Could you check a few things on this model? Use its own coordinates, in mm. A direction names the side the tool comes from. Coordinates: 2 decimals unless noted, no trailing zeros. Write each loop counter-clockwise with the first axis right and the second up, starting at its lowest first coordinate (ties: lowest second). Pieces come first, ordered by that corner, then holes.
```python
from build123d import *

# Parameters (mm, degrees)
ESQUISSE1_R             = 1.5
BOSS_EXTRU_1_DEPTH      = 3
ESQUISSE2_R             = 1.5
ENL_V_MAT_EXTRU_1_DEPTH = 50.779679597
CONG_1_R                = 2


with BuildPart() as part:
    # Esquisse1 → Boss.-Extru.1 (new body)
    with BuildSketch(Plane.XY):
        with BuildLine():
            Line((-22.956336023, 0), (-22.956336023, 5))
            Line((-22.956336023, 5), (-10.956336023, 5))
            Line((-10.956336023, 5), (-10.956336023, 0))
            Line((-10.956336023, 0), (5.043663977, 0))
            Line((5.043663977, 0), (5.043663977, 5))
            Line((5.043663977, 5), (17.043663977, 5))
            Line((17.043663977, 5), (17.043663977, -11))
            Line((17.043663977, -11), (-42.956336023, -11))
            ThreePointArc((-42.956336023, -11), (-48.456336023, -5.5), (-42.956336023, 0))
            Line((-42.956336023, 0), (-22.956336023, 0))
        make_face()
        with Locations((-19.956336023, 2.5)):
            Circle(ESQUISSE1_R, mode=Mode.SUBTRACT)
        with Locations(Location((-13.956336023, 2.5, 0), (0, 0, 180))):
            Circle(ESQUISSE1_R, mode=Mode.SUBTRACT)
        with Locations((8.043663977, 2.5)):
            Circle(ESQUISSE1_R, mode=Mode.SUBTRACT)
        with Locations(Location((14.043663977, 2.5, 0), (0, 0, 180))):
            Circle(ESQUISSE1_R, mode=Mode.SUBTRACT)
    extrude(amount=BOSS_EXTRU_1_DEPTH)

    # Esquisse2 → Enlèv. mat.-Extru.1 (cut, through all)
    with BuildSketch(Plane.XY.offset(3)):
        with Locations((-42.956336023, -5.5)):
            Circle(ESQUISSE2_R)
    extrude(amount=-ENL_V_MAT_EXTRU_1_DEPTH, mode=Mode.SUBTRACT)

    # Congé1
    cong_1_edges = [part.edges().sort_by_distance(p)[0] for p in [
        (-22.956336023, 5, 1.5),
        (-10.956336023, 5, 1.5),
        (5.043663977, 5, 1.5),
        (17.043663977, 5, 1.5),
        (17.043663977, -11, 1.5),
    ]]
    fillet(cong_1_edges, radius=CONG_1_R)


solid = part.part
```
1. I want a section at D-D on x = -35.5. Please give me the cut outline in (y, z), plus the area to 3 significant figures.
Verdict:
outline: (-11, 0) - (0, 0) - (0, 3) - (-11, 3) - close
area: 33.0 mm2
2. I want a section at C-C on x = -43.5. Please give me the cut outline in (y, z).
Verdict:
outline: (-10.97, 0) - (-6.9, 0) - (-6.9, 3) - (-10.97, 3) - close; (-4.1, 0) - (-0.03, 0) - (-0.03, 3) - (-4.1, 3) - close
3. For pin 1 (0.9 mm diameter, centred on x = -4, z = 2, fed in from +Y); pin 2 (1.5 mm diameter, centred on y = 1, z = 1, fed in from -X), each with a flat end and sliding along its axis, tell me the tip position at first contact or that it passes through.
Verdict:
pin 1: stops at y = 0
pin 2: stops at x = -22.96
4. I want a section at A-A on z = 0.7. Please give me the cut outline in (x, y), plus the area to 3 significant figures.
Verdict:
outline: (-42.96, -11) - (15.04, -11) arc R2 ccw to (17.04, -9) - (17.04, 3) arc R2 ccw to (15.04, 5) - (7.04, 5) arc R2 ccw to (5.04, 3) - (5.04, 0) - (-10.96, 0) - (-10.96, 3) arc R2 ccw to (-12.96, 5) - (-20.96, 5) arc R2 ccw to (-22.96, 3) - (-22.96, 0) - (-42.96, 0) arc R5.5 ccw to start; hole circle Ø3 at (-42.96, -5.5); hole circle Ø3 at (-19.96, 2.5); hole circle Ø3 at (-13.96, 2.5); hole circle Ø3 at (8.04, 2.5); hole circle Ø3 at (14.04, 2.5)
area: 788 mm2
5. Please list where these lines run through material, in increasing order: line 1 along X through (y, z) = (0.75, 0.5); line 2 along X through (y, z) = (-6.25, 1.55); line 3 along Y through (x, z) = (-2, 0.15).
Verdict:
line 1: x = -22.96 to -10.96, 5.04 to 17.04
line 2: x = -48.4 to -44.26, -41.66 to 17.04
line 3: y = -11 to 0
6. On a 3-axis mill with a long thin cutter (end or side, diameter ignored), from which of +Z, -Z, +X, -X, +Y, -Y can I reach the whole of each face in a straight line? I mean faces 1 (the face through (11, 5, 1)), 2 (the face through (5.614, 4.399, 1.521)), 3 (the face through (-33, 0, 1)). Say none if no direction works.
Verdict:
face 1: +Z, -Z, +X, -X, +Y
face 2: +Z, -Z, +Y
face 3: +Z, -Z, -X, +Y
7. If we mould it in two halves opening along Y, with no side actions, what happens to faces 4 (the face through (-15.387, 2.049, 1.479)), 5 (the face through (-48.455, -5.621, 1.479)), 6 (the face through (-17, 5, 1))? For each: pulls with the +Y half, pulls with the -Y half, needs draft (parallel to the pull), parting line crosses it, or undercut.
Verdict:
face 4: undercut
face 5: parting line crosses it
face 6: pulls with the +Y half
8. I want a section at B-B on y = -5.5. Please give me the cut outline in (x, z), plus the area to 4 significant figures.
Verdict:
outline: (-48.46, 0) - (-44.46, 0) - (-44.46, 3) - (-48.46, 3) - close; (-41.46, 0) - (17.04, 0) - (17.04, 3) - (-41.46, 3) - close
area: 187.5 mm2
